Check sheet for the modelled part. Datum: model origin and axes. Units: mm. A direction names the side the tool comes from. Coordinates: 2 decimals unless noted, no trailing zeros. Loops run counter-clockwise (first coordinate to the right, second up) from the corner with the lowest first, then second, coordinate; pieces in that order, holes last. Notation, with made-up numbers: M 39,-12 L 95,-12 A10 cw 95,-2 Z; hole C -8,22.5 d1. An arc over 180 degrees is marked long. Write each question's results on one line, items separated by ' | '. Start each with the question number.
from build123d import *

# Parameters (mm, degrees)
SKETCH006_R         = 12.5
PAD001_DEPTH        = 15
SKETCH007_R         = 25
PAD002_DEPTH        = 74
LINEARPATTERN_COUNT = 2
LINEARPATTERN_PITCH = 69
SKETCH008_W         = 252.12847
SKETCH008_H         = 13.500198
POCKET002_DEPTH     = 218.001
SKETCH009_R         = 2.5
HOLE001_DEPTH       = 16
CHAMFER001_SIZE     = 1


with BuildPart() as part:
    # Sketch006 → Pad001 (new body)
    with BuildSketch(Plane.XY):
        with BuildLine():
            ThreePointArc((0, 38), (11.129942, 11.129942), (38, 0))
            Line((38, 0), (180, 0))
            ThreePointArc((180, 0), (215.107422, 23.45803), (206.870058, 64.870058))
            Line((64.870058, 206.870058), (206.870058, 64.870058))
            ThreePointArc((64.870058, 206.870058), (23.45803, 215.107422), (0, 180))
            Line((0, 180), (0, 38))
        make_face()
        with Locations((38, 180)):
            Circle(SKETCH006_R, mode=Mode.SUBTRACT)
        with Locations((180, 38)):
            Circle(SKETCH006_R, mode=Mode.SUBTRACT)
        with Locations((38, 38)):
            Circle(SKETCH006_R, mode=Mode.SUBTRACT)
    pad001 = extrude(amount=PAD001_DEPTH)

    # Sketch007 (on DatumPlane) → Pad002 (join)
    with BuildSketch(Plane.XY.offset(20)):
        with Locations((106, 60)):
            Circle(SKETCH007_R)
    extrude(amount=-PAD002_DEPTH)

    # LinearPattern: Pad001 ×2
    with Locations(*[(0, 0, -i * LINEARPATTERN_PITCH) for i in range(1, LINEARPATTERN_COUNT)]):
        add(pad001)

    # Sketch008 (on DatumPlane) → Pocket002 (cut, through all)
    with BuildSketch(Plane.XZ):
        with Locations((99.729314, -72.750099)):
            Rectangle(SKETCH008_W, SKETCH008_H)
    extrude(amount=-POCKET002_DEPTH, mode=Mode.SUBTRACT)

    # Sketch009 (on Face23 of LinearPattern) → Hole001 (cut)
    with BuildSketch(Plane.XY.offset(15)):
        with Locations((50.325314, 158.249445)):
            Circle(SKETCH009_R)
        with Locations((61.786113, 45.695507)):
            Circle(SKETCH009_R)
        with Locations((156.036591, 45.124257)):
            Circle(SKETCH009_R)
    extrude(amount=-HOLE001_DEPTH, mode=Mode.SUBTRACT)

    # Chamfer001
    chamfer001_edges = [part.edges().sort_by_distance(p)[0] for p in [
        (81, 60, 20),
    ]]
    chamfer(chamfer001_edges, length=CHAMFER001_SIZE)


solid = part.part
1) Gauge pin test, flat ends, axial feed: P1, Ø22.5, axis at x = 180, y = 38, coming from the -Z side; P2, Ø8, axis at x = 85, y = 165.5, coming from the +Z side. Record the tip position at first contact, or that the pin passes through.
2) Section check B-B (y = 99.5). Enter the section's corners in (x, z), then the cut area to 3 significant figures.
3) Set-up check for faces 1 (the cylindrical face through (62.94, 43.478, 7.605)), 2 (the cylindrical face through (28.08, 30.394, 7.395)): record each of +Z, -Z, +X, -X, +Y, -Y from which the full face is reachable in a straight line by a thin tool's end or side.
4) Release check for a two-part mould opening along Z. For faces 3 (the cylindrical face through (87.574, 76.896, -26.622)), 4 (the flat face through (83, 83, -66)), 5 (the cylindrical face through (214.863, 22.881, -60.084)) record: +Z half, -Z half, draft (parallel to the pull), parting line (faces both ways), or undercut.
5) Section check A-A (z = -59). Enter the section's corners in (x, y), then the cut area to 3 significant figures.
6) Thickness scan on probe 1 along X at (y, z) = (38, -62.5); probe 2 along Z at (x, y) = (104, 14); probe 3 along X at (y, z) = (58.5, -19.5). Record the ranges inside material, lowest first.
7) Section check C-C (x = 32). Enter the section's corners in (y, z), then the cut area to 3 significant figures.
8) Section check D-D (x = 106). Enter the section's corners in (y, z).
Return value:
1) P1: passes through | P2: stops at z = 15
2) outline: M 0,-66 L 172.24,-66 L 172.24,-54 L 0,-54 Z; M 0,0 L 172.24,0 L 172.24,15 L 0,15 Z | area: 4,650 mm2
3) face 1: +Z | face 2: +Z, -Z
4) face 3: undercut | face 4: -Z half | face 5: draft
5) outline: M 0,38 A38 ccw 38,0 L 180,0 A38 ccw 206.87,64.87 L 64.87,206.87 A38 ccw 0,180 Z; hole C 38,38 d25; hole C 38,180 d25; hole C 180,38 d25 | area: 31,600 mm2
6) probe 1: x = 0 to 25.5, 50.5 to 167.5, 192.5 to 218 | probe 2: z = -66 to -54, 0 to 15 | probe 3: x = 81.05 to 130.95
7) outline: M 0.48,-66 L 27.03,-66 L 27.03,-54 L 0.48,-54 Z; M 0.48,0 L 27.03,0 L 27.03,15 L 0.48,15 Z; M 48.97,-66 L 169.03,-66 L 169.03,-54 L 48.97,-54 Z; M 48.97,0 L 169.03,0 L 169.03,15 L 48.97,15 Z; M 190.97,-66 L 217.52,-66 L 217.52,-54 L 190.97,-54 Z; M 190.97,0 L 217.52,0 L 217.52,15 L 190.97,15 Z | area: 4,680 mm2
8) outline: M 0,-66 L 165.74,-66 L 165.74,-54 L 85,-54 L 85,0 L 165.74,0 L 165.74,15 L 85,15 L 85,19 L 84,20 L 36,20 L 35,19 L 35,15 L 0,15 L 0,0 L 35,0 L 35,-54 L 0,-54 Z
